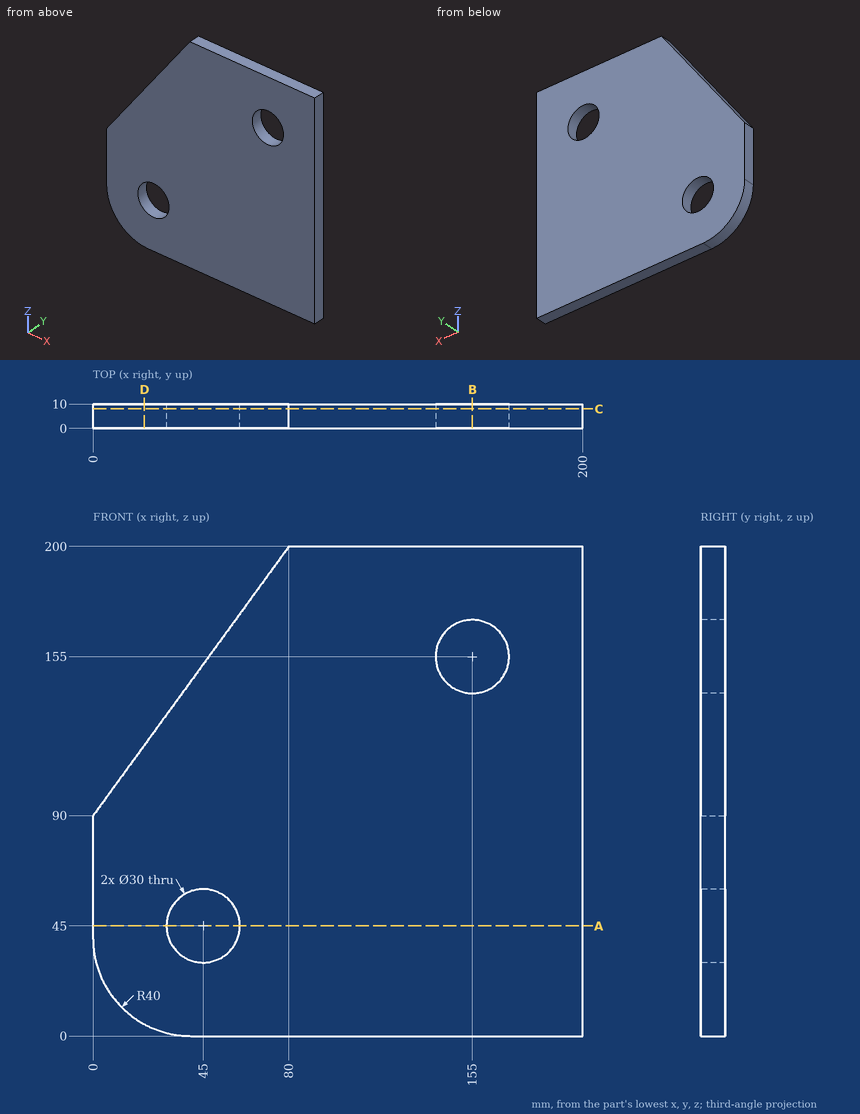
Verification items for this drawing (mm, ordinates from the low corner). Round coordinates to 2 decimals unless told otherwise and drop trailing zeros. Write each loop counter-clockwise with the first axis right and the second up, starting at its lowest first coordinate (ties: lowest second). Pieces come first, ordered by that corner, then holes. Notation, with made-up numbers: (68.5, -36) - (98.5, -36) arc R29 ccw to (98.5, -4) - close; hole circle Ø3 at (-39, 84.25). An arc over 180 degrees is marked (long way). One line per item, written item: value.
1. Cross-section at B-B on x = 155. Record the boundary of the cut face in (y, z).
The answers:
outline: (0, 0) - (10, 0) - (10, 140) - (0, 140) - close; (0, 170) - (10, 170) - (10, 200) - (0, 200) - close
2. Scan lines: L1, parallel to Z at x = 155, y = 3.75; L2, parallel to Z at x = 143, y = 1.25; L3, parallel to X at y = 3.75, z = 158. Record each from-to range of solid material in increasing order.
The answers:
L1: z = 0 to 140, 170 to 200
L2: z = 0 to 146, 164 to 200
L3: x = 49.45 to 140.3, 169.7 to 200
3. Cross-section at A-A on z = 45. Record the boundary of the cut face in (x, y).
The answers:
outline: (0, 0) - (30, 0) - (30, 10) - (0, 10) - close; (60, 0) - (200, 0) - (200, 10) - (60, 10) - close
4. Cross-section at D-D on x = 21. Record the boundary of the cut face in (y, z) (3 decimals), and give its area (3 significant figures).
The answers:
outline: (0, 4.801) - (10, 4.801) - (10, 118.875) - (0, 118.875) - close
area: 1,140 mm^2
5. Depth check by flat-ended pin: pin 1 Ø24 at (x, z) = (155, 155) entering from +Y; pin 2 Ø1.5 at (y, z) = (1, 152.5) entering from -X; pin 3 Ø1 at (y, z) = (6.5, 111) entering from -X. Enter the tip coordinate at first touch or a pass-through.
The answers:
pin 1: passes through
pin 2: stops at x = 44.91
pin 3: stops at x = 14.91
6. Cross-section at C-C on y = 8. Record the boundary of the cut face in (x, z).
The answers:
outline: (0, 40) arc R40 ccw to (40, 0) - (200, 0) - (200, 200) - (80, 200) - (0, 90) - close; hole circle Ø30 at (45, 45); hole circle Ø30 at (155, 155)
